```python
from build123d import *

# Parameters (mm, degrees)
SKETCH1_R           = 90
BOSS_EXTRUDE1_DEPTH = 30
SKETCH2_R           = 80
SKETCH2_R_2         = 45
CUT_EXTRUDE2_DEPTH  = 25
SKETCH3_R           = 35
CUT_EXTRUDE3_DEPTH  = 30
CUT_EXTRUDE6_START  = -5
SKETCH4_R           = 90
SKETCH4_R_2         = 85
CUT_EXTRUDE6_DEPTH  = 5
CUT_EXTRUDE7_DEPTH  = 3
FILLET4_R           = 5
FILLET5_R           = 5
FILLET7_R           = 1
SKETCH8_R           = 45
CUT_EXTRUDE8_DEPTH  = 5


with BuildPart() as part:
    # Sketch1 → Boss-Extrude1 (new body)
    with BuildSketch(Plane(origin=(0, 0, 0), x_dir=(1, 0, 0), z_dir=(0, 1, 0))):
        with Locations(Location((0, 0, 0), (0, 0, 270))):
            Circle(SKETCH1_R)
    extrude(amount=BOSS_EXTRUDE1_DEPTH)

    # Sketch2 → Cut-Extrude2 (cut)
    with BuildSketch(Plane(origin=(0, 30, 0), x_dir=(1, 0, 0), z_dir=(0, 1, 0))):
        with Locations(Location((0, 0, 0), (0, 0, 270))):
            Circle(SKETCH2_R)
        with Locations(Location((0, 0, 0), (0, 0, 270))):
            Circle(SKETCH2_R_2, mode=Mode.SUBTRACT)
    extrude(amount=-CUT_EXTRUDE2_DEPTH, mode=Mode.SUBTRACT)

    # Sketch3 → Cut-Extrude3 (cut)
    with BuildSketch(Plane(origin=(0, 30, 0), x_dir=(1, 0, 0), z_dir=(0, 1, 0))):
        with Locations(Location((0, 0, 0), (0, 0, 270))):
            Circle(SKETCH3_R)
    extrude(amount=-CUT_EXTRUDE3_DEPTH, mode=Mode.SUBTRACT)

    # Sketch4 → Cut-Extrude6 (cut)
    with BuildSketch(Plane(origin=(0, 30, 0), x_dir=(1, 0, 0), z_dir=(0, 1, 0)).offset(CUT_EXTRUDE6_START)):
        with Locations(Location((0, 0, 0), (0, 0, 270))):
            Circle(SKETCH4_R)
        with Locations(Location((0, 0, 0), (0, 0, 270))):
            Circle(SKETCH4_R_2, mode=Mode.SUBTRACT)
    extrude(amount=CUT_EXTRUDE6_DEPTH, mode=Mode.SUBTRACT)

    # Sketch7 → Cut-Extrude7 (cut)
    with BuildSketch(Plane(origin=(0, 0, 0), x_dir=(-1, 0, 0), z_dir=(0, -1, 0))):
        Polygon((-43.33470773, 87.639434023), (16.290699143, -18.176389433), (7.60290089, -23.128375045), (-52.007029161, 82.661204336), align=None)
    extrude(amount=-CUT_EXTRUDE7_DEPTH, mode=Mode.SUBTRACT)

    # Fillet4
    # the kernel refuses this fillet: 5 mm, written as the material it adds along each edge
    with BuildSketch(Plane(origin=(15.521035458, 3, -17.909611373), x_dir=(0, -1, 0), z_dir=(0.490907288805725, 0, -0.871211819133219))) as fillet4_piece_1_section:
        with BuildLine():
            CenterArc((5, 4.582575695), FILLET4_R, 180, 66.421821522)
            Line((0, 4.582575695), (-0.1, 4.582575695))
            Line((-0.1, 4.582575695), (-0.1, 0))
            Line((-0.1, 0), (0, -0.1))
            ThreePointArc((0, -0.1), (1.5, -0.1), (2.96, -0.091651514))
            Line((2.96, -0.091651514), (3, 0))
        make_face()
    fillet4_piece_1 = extrude(amount=78.109596927, mode=Mode.PRIVATE)
    fillet4_piece_1 = fillet4_piece_1 & Plane(origin=(0, 3, 0), x_dir=(0, 0, 1), z_dir=(0, -1, 0)) * Cylinder(90, 175, mode=Mode.PRIVATE)
    fillet4_piece_1 = fillet4_piece_1 - Plane(origin=(0, 3, 0), x_dir=(0, 0, 1), z_dir=(0, 1, 0)) * Cylinder(35, 175, mode=Mode.PRIVATE)
    add(fillet4_piece_1)

    # Fillet5
    # the kernel refuses this fillet: 5 mm, written as the material it adds along each edge
    with BuildSketch(Plane(origin=(45.139410265, 3, -90.842197657), x_dir=(0.8712093933197586, 0, 0.4909115938653498), z_dir=(-0.4909115938653499, 0, 0.8712093933197586))) as fillet5_piece_1_section:
        with BuildLine():
            CenterArc((4.582575695, -5), FILLET5_R, 90, 66.421821522)
            Line((0, -3), (-0.091651514, -2.96))
            ThreePointArc((-0.091651514, -2.96), (-0.1, -1.5), (-0.1, 0))
            Line((-0.1, 0), (0, 0.1))
            Line((0, 0.1), (4.582575695, 0.1))
            Line((4.582575695, 0.1), (4.582575695, 0))
        make_face()
    fillet5_piece_1 = extrude(amount=78.15744592, mode=Mode.PRIVATE)
    fillet5_piece_1 = fillet5_piece_1 - Plane(origin=(0, 3, 0), x_dir=(0, 0, 1), z_dir=(0, 1, 0)) * Cylinder(35, 175, mode=Mode.PRIVATE)
    fillet5_piece_1 = fillet5_piece_1 & Plane(origin=(0, 3, 0), x_dir=(0, 0, 1), z_dir=(0, -1, 0)) * Cylinder(90, 175, mode=Mode.PRIVATE)
    add(fillet5_piece_1)

    # Fillet6: read off the stored shape, not the designer's step
    # Fillet6 outline → Fillet6 (revolve, cut)
    with BuildSketch(Plane.XY):
        with BuildLine():
            ThreePointArc((90, 1), (89.707106781, 0.292893219), (89, 0))
            Line((89, 0), (90, 0))
            Line((90, 0), (90, 1))
        make_face()
    revolve(axis=Axis((0, 0, 0), (0, 1, 0)), mode=Mode.SUBTRACT)

    # Fillet7
    fillet7_edges = [part.edges().sort_by_distance(p)[0] for p in [
        (0, 30, -85),
    ]]
    fillet(fillet7_edges, radius=FILLET7_R)

    # Sketch8 → Cut-Extrude8 (cut)
    with BuildSketch(Plane(origin=(0, 30, 0), x_dir=(1, 0, 0), z_dir=(0, 1, 0))):
        with Locations(Location((0, 0, 0), (0, 0, 270))):
            Circle(SKETCH8_R)
    extrude(amount=-CUT_EXTRUDE8_DEPTH, mode=Mode.SUBTRACT)


solid = part.part
```
The model under review builds one solid part; all positions refer to its coordinate system, in mm. A direction names the side the tool comes from. Give positions to 0.01 mm unless a question says otherwise; leave off trailing zeros. Write each loop counter-clockwise with the first axis right and the second up, starting at its lowest first coordinate (ties: lowest second). Pieces come first, ordered by that corner, then holes.
(1) The part is to be moulded in two halves that separate along Z. For faces 1 (the cylindrical face through (27.819, 2.205, -56.278)), 2 (the cylindrical face through (-34.471, 12.832, 83.137)), 3 (the flat face through (54, 25, 66)), say which applies: released by +Z, released by -Z, zero draft, split by the parting line, or undercut.
(2) Consider section B-B, the plane z = 0. Give the boundary of the cut face in (x, y).
(3) To check wall thickness, follow L1, parallel to X at y = 9, z = 0; L2, parallel to X at y = 8.5, z = 38; L3, parallel to X at y = 10.5, z = -2 (3 decimals). State the ranges of each line that lie inside material, in increasing order.
(4) Consider section C-C, the plane y = 13. Give the boundary of the cut face in (x, z).
(5) Tool access review of faces 4 (the cylindrical face through (32.898, 2.205, -52.573)), 5 (the cylindrical face through (-21, 13, -28)), 6 (the flat face through (-26.5, 25, 23.1)): name each direction out of +Z, -Z, +X, -X, +Y, -Y from which nothing blocks a thin tool from reaching the whole face with its end or side.
(6) For P1, Ø2, axis at x = -17.5, z = -71.5, coming from the +Y side; P2, Ø8, axis at x = 25.5, z = 19.5, coming from the +Y side; P3, Ø3, axis at y = 14, z = 35.5, coming from the -X side, all flat-tipped, find the tip position at first contact; note any pin that passes through.
(7) Consider section A-A, the plane x = 0. Give the boundary of the cut face in (y, z).
Returned:
1. face 1: undercut
1. face 2: split by the parting line
1. face 3: zero draft
2. outline: (-90, 1) arc R1 ccw to (-89, 0) - (-35, 0) - (-35, 25) - (-45, 25) - (-45, 5) - (-80, 5) - (-80, 30) - (-84, 30) arc R1 ccw to (-85, 29) - (-85, 25) - (-90, 25) - close; (35, 0) - (89, 0) arc R1 ccw to (90, 1) - (90, 25) - (85, 25) - (85, 29) arc R1 ccw to (84, 30) - (80, 30) - (80, 5) - (45, 5) - (45, 25) - (35, 25) - close
3. L1: x = -90 to -80, -45 to -35, 35 to 45, 80 to 90
3. L2: x = -81.58 to -70.4, -24.1 to 24.1, 70.4 to 81.58
3. L3: x = -89.978 to -79.975, -44.956 to -34.943, 34.943 to 44.956, 79.975 to 89.978
4. outline: circle Ø180 at (0, 0); circle Ø90 at (0, 0); hole circle Ø160 at (0, 0); hole circle Ø70 at (0, 0)
5. face 4: -Y
5. face 5: +Y, -Y
5. face 6: +Y
6. P1: stops at y = 5
6. P2: stops at y = 25
6. P3: stops at x = -83.33
7. outline: (0, -89) arc R1 ccw to (1, -90) - (25, -90) - (25, -85) - (29, -85) arc R1 ccw to (30, -84) - (30, -80) - (5, -80) - (5, -45) - (25, -45) - (25, -35) - (0, -35) - close; (0, 35) - (25, 35) - (25, 45) - (5, 45) - (5, 80) - (30, 80) - (30, 84) arc R1 ccw to (29, 85) - (25, 85) - (25, 90) - (1, 90) arc R1 ccw to (0, 89) - close
